Check sheet for the drawn part. Datum: minimum x, y, z corner. Units: mm. A direction names the side the tool comes from. Round coordinates to 2 decimals unless told otherwise and drop trailing zeros. Write each loop counter-clockwise with the first axis right and the second up, starting at its lowest first coordinate (ties: lowest second). Pieces come first, ordered by that corner, then holes. Notation, with made-up numbers: M 87.5,18 L 115.5,18 A19 cw 115.5,41 Z; hole C 32,64.25 d8. An arc over 180 degrees is marked long. Use a Markdown table: item, result.
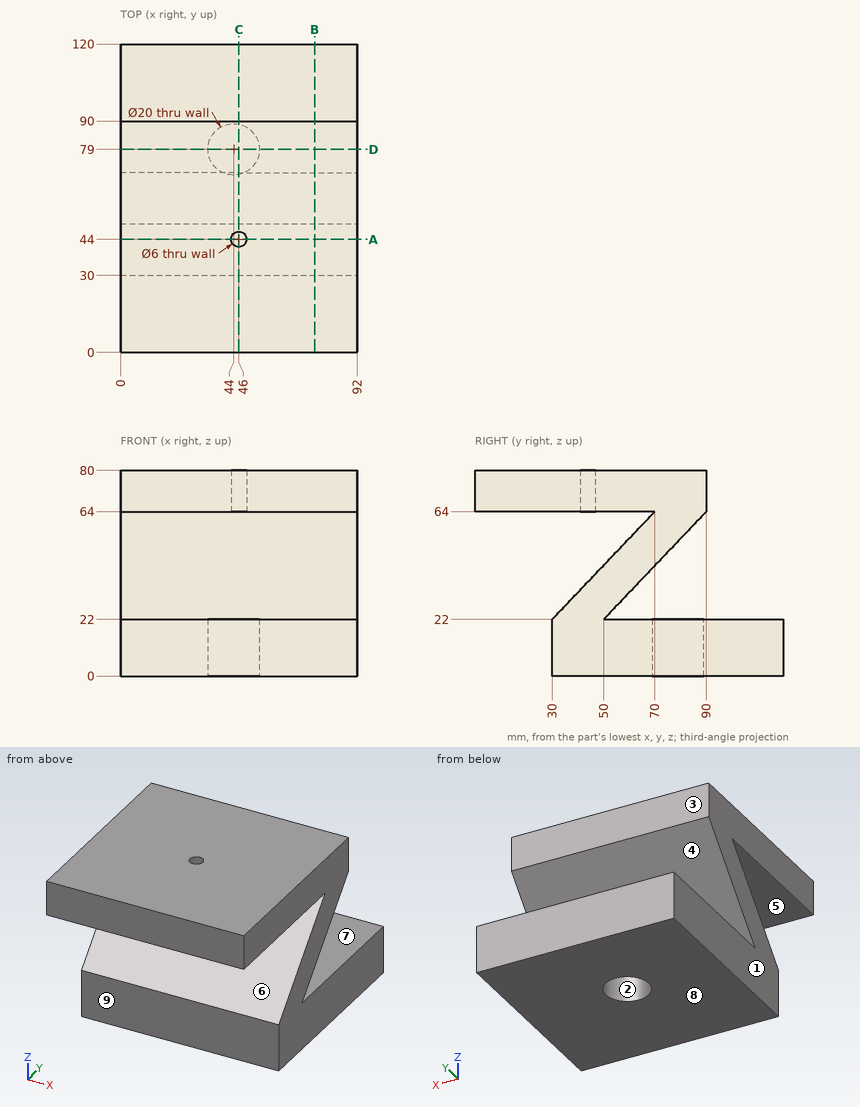
Item 1: Access from +Z, -Z, +X, -X, +Y, -Y to the whole of each face (thin tool, end or side, straight path). Record for the marked faces 1, 2, 3, 4 and 5.
Outcome:
| item | result |
|---|---|
| face 1 | +Z, -Z, -X, +Y, -Y |
| face 2 | -Z |
| face 3 | +Z, +X, -X, +Y |
| face 4 | +X, -X, +Y |
| face 5 | +X, -X, -Y |
Item 2: Cross-section at C-C, the plane x = 46. Record the cut outline in (y, z).
Outcome:
| item | result |
|---|---|
| outline | M 0,64 L 41,64 L 41,80 L 0,80 Z; M 30,0 L 69.2,0 L 69.2,22 L 50,22 L 90,64 L 90,80 L 47,80 L 47,64 L 70,64 L 30,22 Z; M 88.8,0 L 120,0 L 120,22 L 88.8,22 Z |
Item 3: Go/stop test with flat-tipped pins: pin 1 (1.5 mm diameter, centred on x = 24.5, z = 61, fed in from +Y); pin 2 (10 mm diameter, centred on x = 50.5, y = 106.5, fed in from +Z); pin 3 (5 mm diameter, centred on x = 46, y = 44, fed in from +Z) (3 decimals). Record where each tip stops, or that it passes through.
Outcome:
| item | result |
|---|---|
| pin 1 | stops at y = 87.86 |
| pin 2 | stops at z = 22 |
| pin 3 | stops at z = 39.325 |
Item 4: Material ranges on line 1 along X through (y, z) = (79, 14.75); line 2 along Z through (x, y) = (26, 64); line 3 along Z through (x, y) = (88.5, 61.5) (3 decimals), recorded low to high. Write a range as from..to.
Outcome:
| item | result |
|---|---|
| line 1 | x = 0..34, 54..92 |
| line 2 | z = 0..22, 36.7..57.7, 64..80 |
| line 3 | z = 0..22, 34.075..55.075, 64..80 |
Item 5: Cross-section at D-D, the plane y = 79. Record the cut outline in (x, z), and give its area (3 significant figures).
Outcome:
| item | result |
|---|---|
| outline | M 0,0 L 34,0 L 34,22 L 0,22 Z; M 0,52.45 L 92,52.45 L 92,80 L 0,80 Z; M 54,0 L 92,0 L 92,22 L 54,22 Z |
| area | 4,120 mm2 |
Item 6: Mould release check, pull along Z, two halves, no side actions. Record for the marked faces 6, 7, 8 and 9: +Z half, -Z half, draft (parallel to the pull), parting line (faces both ways), or undercut.
Outcome:
| item | result |
|---|---|
| face 6 | undercut |
| face 7 | undercut |
| face 8 | -Z half |
| face 9 | draft |
Item 7: Cross-section at A-A, the plane y = 44. Record the cut outline in (x, z), and give its area (3 significant figures).
Outcome:
| item | result |
|---|---|
| outline | M 0,0 L 92,0 L 92,36.7 L 0,36.7 Z; M 0,64 L 43,64 L 43,80 L 0,80 Z; M 49,64 L 92,64 L 92,80 L 49,80 Z |
| area | 4,750 mm2 |
Item 8: Cross-section at B-B, the plane x = 75.5. Record the cut outline in (y, z).
Outcome:
| item | result |
|---|---|
| outline | M 0,64 L 70,64 L 30,22 L 30,0 L 120,0 L 120,22 L 50,22 L 90,64 L 90,80 L 0,80 Z |
